from build123d import *

# Parameters (mm, degrees)
SKETCH1_R               = 7.9375
SKETCH1_R_2             = 3.96875
BOSS_EXTRUDE1_DEPTH     = 9.525
CUT_EXTRUDE1_DEPTH      = 15.721869362
CUT_EXTRUDE1_DEPTH_BACK = 15.721869362


with BuildPart() as part:
    # Sketch1 → Boss-Extrude1 (new body)
    with BuildSketch(Plane(origin=(0, 0, 0), x_dir=(1, 0, 0), z_dir=(0, 1, 0))):
        with Locations(Location((0, 0, 0), (0, 0, 90))):
            Circle(SKETCH1_R)
        with Locations(Location((0, 0, 0), (0, 0, 90))):
            Circle(SKETCH1_R_2, mode=Mode.SUBTRACT)
    extrude(amount=BOSS_EXTRUDE1_DEPTH)

    # Sketch2 → Cut-Extrude1 (cut, two sides: drawn at the far end of the back side and taken through both)
    with BuildSketch(Plane(origin=(0, 0, 0), x_dir=(0, 0, -1), z_dir=(1, 0, 0)).offset(-CUT_EXTRUDE1_DEPTH_BACK)):
        with BuildLine():
            Line((-4.7625, 9.525), (4.7625, 9.525))
            Line((4.7625, 9.525), (4.7625, 7.14375))
            ThreePointArc((4.7625, 7.14375), (4.113428058, 5.508074192), (2.519424024, 4.7625))
            Line((2.519424024, 4.7625), (-2.38125, 4.7625))
            ThreePointArc((-2.38125, 4.7625), (-4.065048023, 5.459951977), (-4.7625, 7.14375))
            Line((-4.7625, 7.14375), (-4.7625, 9.525))
        make_face()
    extrude(amount=CUT_EXTRUDE1_DEPTH + CUT_EXTRUDE1_DEPTH_BACK, mode=Mode.SUBTRACT)


solid = part.part
Input: part model. Units: mm. Frame: model coordinates. A direction names the side the tool comes from. Coordinates: 2 decimals unless noted, no trailing zeros. Order: outer loops, then holes, each group sorted by start corner. A loop starts at its lowest first (then second) coordinate and runs counter-clockwise, first axis right, second up.
1. Access query for faces 4 (the cylindrical face through (1.52, 2.647, -3.666)), 5 (the cylindrical face through (-0.105, 5.527, -4.131)). Directions: +Z, -Z, +X, -X, +Y, -Y. A direction counts if a zero-diameter tool reaches every point of the face in a straight line with its end or side. Return the directions, or none.
Checked values:
face 4: +Y, -Y
face 5: +X, -X, +Y
2. Contact query for flat-ended pins moving along their axis: P1, Ø4, axis at x = 3.5, y = 8.5, coming from the -Z side; P2, Ø1.9, axis at x = -3, y = 8.5, coming from the +Z side; P3, Ø5.5, axis at x = -5, z = 0.5, coming from the +Y side. Output: stop coordinate, or through.
Checked values:
P1: stops at z = -7.79
P2: stops at z = 7.67
P3: stops at y = 4.93
3. Draft query along Z for faces 1 (the flat face through (-6, 4.762, 0)), 2 (the cylindrical face through (-0.35, 3.64, 7.93)), 3 (the flat face through (0, 9.525, -6)). Return one class per face: +Z half, -Z half, draft (parallel to the pull), parting line (faces both ways), or undercut.
Checked values:
face 1: undercut
face 2: parting line
face 3: draft
4. Cut plane B-B, the plane x = 1. Return loops of the section in (y, z) (1 decimal).
Checked values:
outline: (0, -7.9) - (9.5, -7.9) - (9.5, -4.8) - (7.1, -4.8) arc R2.4 cw to (5.3, -3.8) - (0, -3.8) - close; (0, 3.8) - (5.3, 3.8) arc R2.4 cw to (7.1, 4.8) - (9.5, 4.8) - (9.5, 7.9) - (0, 7.9) - close
5. Cut plane C-C, the plane y = 3. Return loops of the section in (x, z) (1 decimal).
Checked values:
outline: circle Ø15.9 at (0, 0); hole circle Ø7.9 at (0, 0)
6. Ray query, line 1 along X through (y, z) = (3.2, 0); line 2 along Y through (x, z) = (6.25, -0.5); line 3 along Z through (x, y) = (2.75, 7.5). Return the intervals inside material, ascending.
Checked values:
line 1: x = -7.94 to -3.97, 3.97 to 7.94
line 2: y = 0 to 4.76
line 3: z = -7.45 to -4.76, 4.76 to 7.45
7. Cut plane A-A, the plane z = 0. Return loops of the section in (x, y), plus the area to 3 significant figures.
Checked values:
outline: (-7.94, 0) - (-3.97, 0) - (-3.97, 4.76) - (-7.94, 4.76) - close; (3.97, 0) - (7.94, 0) - (7.94, 4.76) - (3.97, 4.76) - close
area: 37.8 mm2
